Check sheet for the drawn part. Datum: minimum x, y, z corner. Units: mm. Round coordinates to 2 decimals unless told otherwise and drop trailing zeros. Write each loop counter-clockwise with the first axis right and the second up, starting at its lowest first coordinate (ties: lowest second). Pieces come first, ordered by that corner, then holes. Notation, with made-up numbers: (7.5, 19) - (64.5, 19) arc R12 cw to (64.5, 32) - close; hole circle Ø6 at (17, -5.75). An arc over 180 degrees is marked (long way). Return JSON: item names as keys, results as strings. Group by question number.
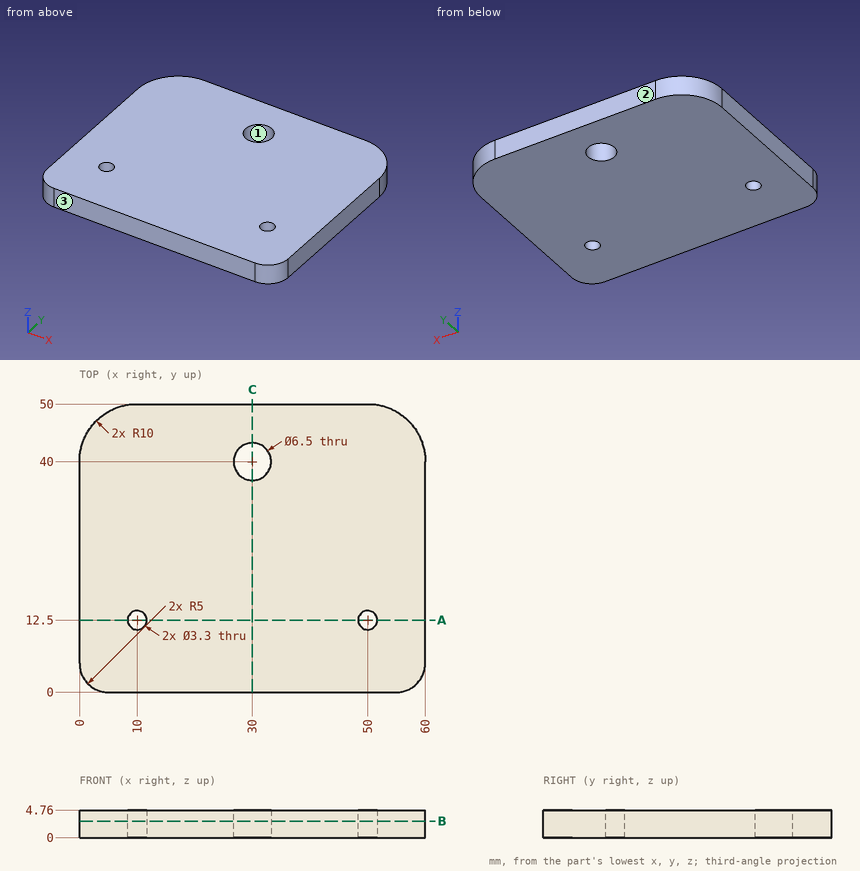
1. Material ranges on line 1 along Y through (x, z) = (30, 1.4); line 2 along Y through (x, z) = (10, 1.25); line 3 along X through (y, z) = (42, 3.85), recorded low to high.
2. Section check C-C (x = 30). Enter the section's corners in (y, z), and give its area (3 significant figures).
3. Section check B-B (z = 2.85). Enter the section's corners in (x, y), and give its area (3 significant figures).
4. Mould release check, pull along Y, two halves, no side actions. Record for the marked faces 1, 2 and 3: pulls with the +Y half, pulls with the -Y half, needs draft (parallel to the pull), parting line crosses it, or undercut.
5. Section check A-A (y = 12.5). Enter the section's corners in (x, z), and give its area (3 significant figures).
6. Depth check by flat-ended pin: pin 1 Ø10.5 at (x, y) = (30, 40) entering from +Z; pin 2 Ø2 at (x, y) = (50, 12.5) entering from +Z. Enter the tip coordinate at first touch or a pass-through.
Result sheet:
{
 "1": {"line 1": "y = 0 to 36.75, 43.25 to 50", "line 2": "y = 0 to 10.85, 14.15 to 50", "line 3": "x = 0.2 to 27.44, 32.56 to 59.8"},
 "2": {"outline": "(0, 0) - (36.75, 0) - (36.75, 4.76) - (0, 4.76) - close; (43.25, 0) - (50, 0) - (50, 4.76) - (43.25, 4.76) - close", "area": "207 mm²"},
 "3": {"outline": "(0, 5) arc R5 ccw to (5, 0) - (55, 0) arc R5 ccw to (60, 5) - (60, 40) arc R10 ccw to (50, 50) - (10, 50) arc R10 ccw to (0, 40) - close; hole circle Ø3.3 at (10, 12.5); hole circle Ø6.5 at (30, 40); hole circle Ø3.3 at (50, 12.5)", "area": "2,900 mm²"},
 "4": {"face 1": "undercut", "face 2": "pulls with the +Y half", "face 3": "pulls with the -Y half"},
 "5": {"outline": "(0, 0) - (8.35, 0) - (8.35, 4.76) - (0, 4.76) - close; (11.65, 0) - (48.35, 0) - (48.35, 4.76) - (11.65, 4.76) - close; (51.65, 0) - (60, 0) - (60, 4.76) - (51.65, 4.76) - close", "area": "254 mm²"},
 "6": {"pin 1": "stops at z = 4.76", "pin 2": "passes through"}
}
